The figure shows three views and two pictorial views of one solid part (mm, origin at its lowest corner). Answer the questions. Coordinates: 2 decimals unless noted, no trailing zeros. Loops run counter-clockwise (first coordinate to the right, second up) from the corner with the lowest first, then second, coordinate; pieces in that order, holes last.
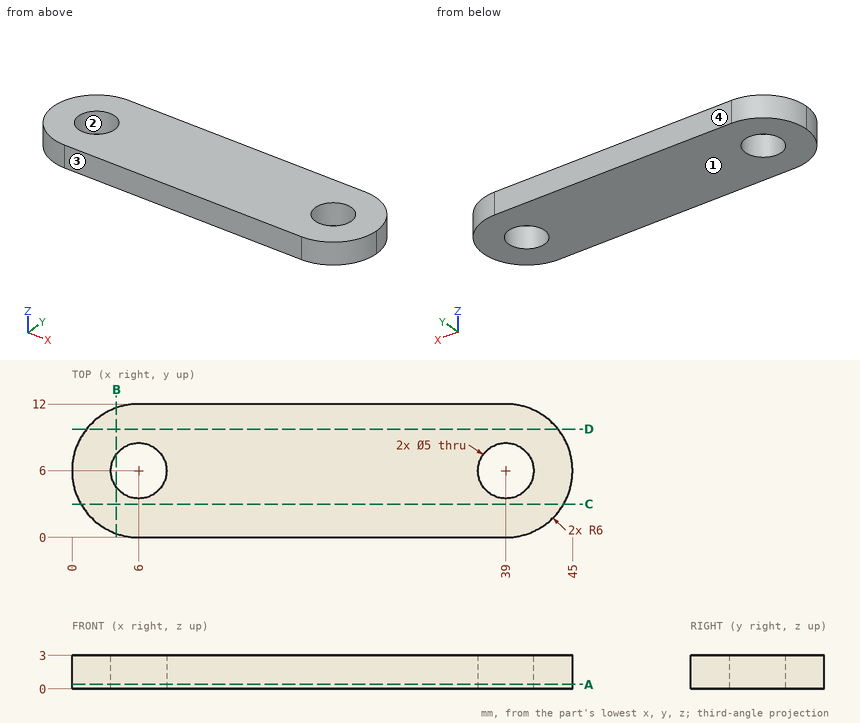
Q1. Determine the mould class of the marked faces 1, 2, 3 and 4 for opening direction Y: +Y half, -Y half, draft (parallel to the pull), parting line (faces both ways), or undercut.
Findings below:
face 1: draft
face 2: undercut
face 3: -Y half
face 4: +Y half
Q2. A cutting plane is placed at C-C (y = 3). Give the vertices of the cut face in (x, z), then the cut area to 3 significant figures.
Findings below:
outline: (0.8, 0) - (44.2, 0) - (44.2, 3) - (0.8, 3) - close
area: 130 mm2
Q3. A flat-ended cylindrical pin translates along its axis: pin 1 Ø5 at (x, y) = (5, 8.5) entering from -Z. Find the tip coordinate at first contact, or state that the pin passes through.
Findings below:
pin 1: stops at z = 0
Q4. A cutting plane is placed at A-A (z = 0.4). Give the vertices of the cut face in (x, y).
Findings below:
outline: (6, 0) - (39, 0) arc R6 ccw to (39, 12) - (6, 12) arc R6 ccw to start; hole circle Ø5 at (6, 6); hole circle Ø5 at (39, 6)
Q5. A cutting plane is placed at D-D (y = 9.75). Give the vertices of the cut face in (x, z), then the cut area to 3 significant figures.
Findings below:
outline: (1.32, 0) - (43.68, 0) - (43.68, 3) - (1.32, 3) - close
area: 127 mm2
Q6. A cutting plane is placed at B-B (x = 4). Give the vertices of the cut face in (y, z).
Findings below:
outline: (0.34, 0) - (4.5, 0) - (4.5, 3) - (0.34, 3) - close; (7.5, 0) - (11.66, 0) - (11.66, 3) - (7.5, 3) - close
Q7. Straight lines are drawn through the part: probe 1 along Y at (x, z) = (39, 2.2); probe 2 along Y at (x, z) = (5, 1.1); probe 3 along X at (y, z) = (2.25, 2.4). For each, find the intervals that lie inside material, in ascending order.
Findings below:
probe 1: y = 0 to 3.5, 8.5 to 12
probe 2: y = 0.08 to 3.71, 8.29 to 11.92
probe 3: x = 1.32 to 43.68
